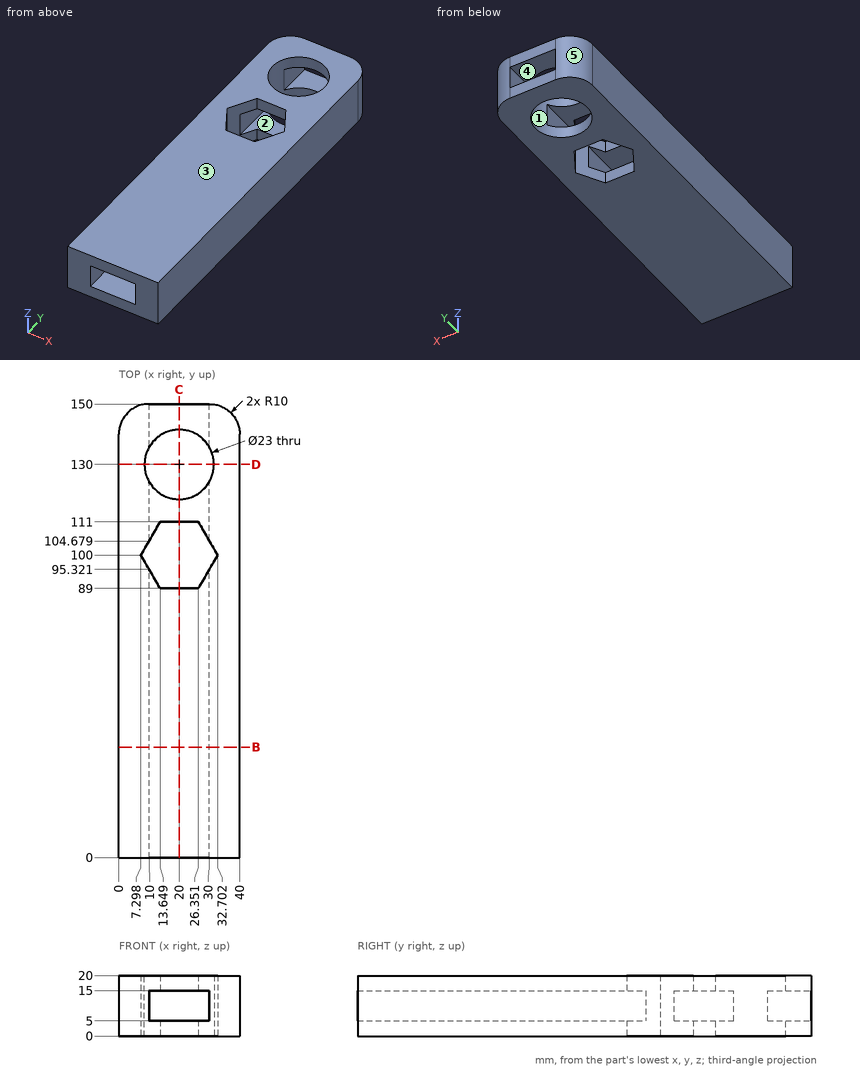
Answer from the drawing. Dimensions are ordinates in mm from the lowest x, y and z of the part. A direction names the side the tool comes from. Round coordinates to 2 decimals unless told otherwise and drop trailing zeros. Loops run counter-clockwise (first coordinate to the right, second up) from the corner with the lowest first, then second, coordinate; pieces in that order, holes last.
(1) Find the intervals of material crossed by L1, parallel to Y at x = 20, z = 4; L2, parallel to Z at x = 12, y = 119; L3, parallel to X at y = 122, z = 10.75, in increasing order.
Computed values:
L1: y = 0 to 89, 111 to 118.5, 141.5 to 150
L2: z = 0 to 5, 15 to 20
L3: x = 0 to 10, 30 to 40
(2) The part is cut by section C-C, the plane x = 20. Give the vertices of the cut face in (y, z), and give its area (3 significant figures).
Computed values:
outline: (0, 0) - (89, 0) - (89, 5) - (0, 5) - close; (0, 15) - (89, 15) - (89, 20) - (0, 20) - close; (111, 0) - (118.5, 0) - (118.5, 5) - (111, 5) - close; (111, 15) - (118.5, 15) - (118.5, 20) - (111, 20) - close; (141.5, 0) - (150, 0) - (150, 5) - (141.5, 5) - close; (141.5, 15) - (150, 15) - (150, 20) - (141.5, 20) - close
area: 1,050 mm2
(3) This flat-tipped pin is pushed along its axis until it touches: P1, Ø6, axis at x = 35.5, z = 8.5, coming from the +Y side. Where does it stop, or does it pass through?
Computed values:
P1: stops at y = 149.68
(4) The part is cut by section D-D, the plane y = 130. Give the vertices of the cut face in (x, z).
Computed values:
outline: (0, 0) - (8.5, 0) - (8.5, 20) - (0, 20) - close; (31.5, 0) - (40, 0) - (40, 20) - (31.5, 20) - close
(5) The mould has two halves that part along X. Classify the marked faces 3, 4 and 5: pulls with the +X half, pulls with the -X half, needs draft (parallel to the pull), parting line crosses it, or undercut.
Computed values:
face 3: needs draft
face 4: undercut
face 5: pulls with the -X half
(6) The part is cut by section B-B, the plane y = 36.5. Give the vertices of the cut face in (x, z).
Computed values:
outline: (0, 0) - (40, 0) - (40, 20) - (0, 20) - close; hole (10, 5) - (30, 5) - (30, 15) - (10, 15) - close
(7) For the marked faces 1 and 2, determine the directions among +Z, -Z, +X, -X, +Y, -Y from which every point of the face is accessible in a straight line to the end or side of a thin tool.
Computed values:
face 1: +Z, -Z
face 2: +Y, -Y
